from build123d import *

# Parameters (mm, degrees)
BOSS_EXTRUDE1_DEPTH          = 19.05
SKETCH7_R                    = 7.62
CUT_EXTRUDE2_DEPTH           = 38.1
SKETCH2_R                    = 11.176
CUT_EXTRUDE1_DEPTH           = 7.239
SKETCH8_R                    = 11.176
CUT_EXTRUDE3_DEPTH           = 7.239
F_10_0_1935_DIAMETER_HOLE1_D = 4.9149


with BuildPart() as part:
    # Sketch1 → Boss-Extrude1 (new body, symmetric)
    with BuildSketch(Plane.XY):
        Polygon((13.335, 25.4), (-13.335, 25.4), (-13.335, 38.1), (-20.447, 38.1), (-20.447, -71.12), (20.447, -71.12), (20.447, 38.1), (13.335, 38.1), align=None)
    extrude(amount=BOSS_EXTRUDE1_DEPTH, both=True)

    # Sketch7 → Cut-Extrude2 (cut)
    with BuildSketch(Plane.XY.offset(19.05)):
        Circle(SKETCH7_R)
        with Locations((0, -50.8)):
            Circle(SKETCH7_R)
    extrude(amount=-CUT_EXTRUDE2_DEPTH, mode=Mode.SUBTRACT)

    # Sketch2 → Cut-Extrude1 (cut)
    with BuildSketch(Plane.XY.offset(19.05)):
        Circle(SKETCH2_R)
        with Locations((0, -50.8)):
            Circle(SKETCH2_R)
    extrude(amount=-CUT_EXTRUDE1_DEPTH, mode=Mode.SUBTRACT)

    # Sketch8 → Cut-Extrude3 (cut)
    with BuildSketch(Plane.XY.offset(-19.05)):
        Circle(SKETCH8_R)
        with Locations((0, -50.8)):
            Circle(SKETCH8_R)
    extrude(amount=CUT_EXTRUDE3_DEPTH, mode=Mode.SUBTRACT)

    # #10 (0.1935) Diameter Hole1 (through all)
    with Locations(Plane(origin=(20.447, 0, 0), x_dir=(0, 0, -1), z_dir=(1, 0, 0))):
        with Locations((-11.43, 31.75)):
            f_10_0_1935_diameter_hole1 = Hole(F_10_0_1935_DIAMETER_HOLE1_D / 2)

    # Mirror1: #10 (0.1935) Diameter Hole1 across plane
    add(f_10_0_1935_diameter_hole1.mirror(Plane.XY), mode=Mode.SUBTRACT)


solid = part.part
For this review, take the finished solid that the model builds, in its own axes (mm). A direction names the side the tool comes from. Give positions to 0.01 mm unless a question says otherwise; leave off trailing zeros. Loops run counter-clockwise (first coordinate to the right, second up) from the corner with the lowest first, then second, coordinate; pieces in that order, holes last.
Item 1: Take a section at B-B, the plane z = -15.5. State the section outline as (x, y) points (3 decimals), and give its area (3 significant figures).
Item 2: Take a section at D-D, the plane y = 31.75. State the section outline as (x, z) points (3 decimals).
Item 3: Tool access review of faces 1 (the flat face through (0, -16, -19.05)), 2 (the cylindrical face through (-16.94, 33.41, -9.62)), 3 (the cylindrical face through (-1.45, -39.72, -15.48)), 4 (the cylindrical face through (-8.87, -6.8, 15.48)), 5 (the flat face through (-13.335, 32, 0)): name each direction out of +Z, -Z, +X, -X, +Y, -Y from which nothing blocks a thin tool from reaching the whole face with its end or side.
Item 4: Take a section at C-C, the plane y = -50.8. State the section outline as (x, z) points.
Item 5: For line 1 along Y through (x, z) = (0, -15.25); line 2 along Y through (x, z) = (18, 11.43); line 3 along X through (y, z) = (26, 16) (3 decimals), list the stretches that pass through material, from the lowest coordinate up.
Item 6: Draft analysis for pull direction Z (two halves, no side actions). For faces 6 (the flat face through (5, -7, 11.811)), 7 (the flat face through (-17, 38.1, 0)), 8 (the cylindrical face through (16.84, 33.41, 9.62)), state which applies: +Z half, -Z half, draft (parallel to the pull), parting line (faces both ways), or undercut.
Item 7: Insertion check: pin 1 (20 mm diameter, centred on x = 0, y = -50.8, fed in from -Z); pin 2 (4.5 mm diameter, centred on y = 31.75, z = 11.43, fed in from +X); pin 3 (21.5 mm diameter, centred on x = 2.5, z = -1.5, fed in from +Y); pin 4 (11 mm diameter, centred on x = -5, y = 1.5, fed in from +Z). Each pin has a flat end and moves straight along its axis. Give the tip position at first contact, or say it passes through.
Item 8: Take a section at A-A, the plane x = 0. State the section outline as (y, z) points, and give its area (3 significant figures).
Calculated:
1. outline: (-20.447, -71.12) - (20.447, -71.12) - (20.447, 38.1) - (13.335, 38.1) - (13.335, 25.4) - (-13.335, 25.4) - (-13.335, 38.1) - (-20.447, 38.1) - close; hole circle Ø22.352 at (0, -50.8); hole circle Ø22.352 at (0, 0)
1. area: 3,340 mm2
2. outline: (-20.447, -19.05) - (-13.335, -19.05) - (-13.335, -13.887) - (-20.447, -13.887) - close; (-20.447, -8.973) - (-13.335, -8.973) - (-13.335, 8.973) - (-20.447, 8.973) - close; (-20.447, 13.887) - (-13.335, 13.887) - (-13.335, 19.05) - (-20.447, 19.05) - close; (13.335, -19.05) - (20.447, -19.05) - (20.447, -13.887) - (13.335, -13.887) - close; (13.335, -8.973) - (20.447, -8.973) - (20.447, 8.973) - (13.335, 8.973) - close; (13.335, 13.887) - (20.447, 13.887) - (20.447, 19.05) - (13.335, 19.05) - close
3. face 1: -Z, +X, -X, +Y, -Y
3. face 2: +X, -X
3. face 3: -Z
3. face 4: +Z
3. face 5: +Z, -Z, +Y
4. outline: (-20.45, -19.05) - (-11.18, -19.05) - (-11.18, -11.81) - (-7.62, -11.81) - (-7.62, 11.81) - (-11.18, 11.81) - (-11.18, 19.05) - (-20.45, 19.05) - close; (7.62, -11.81) - (11.18, -11.81) - (11.18, -19.05) - (20.45, -19.05) - (20.45, 19.05) - (11.18, 19.05) - (11.18, 11.81) - (7.62, 11.81) - close
5. line 1: y = -71.12 to -61.98, -39.62 to -11.18, 11.18 to 25.4
5. line 2: y = -71.12 to 29.29, 34.21 to 38.1
5. line 3: x = -20.447 to -13.335, 13.335 to 20.447
6. face 6: +Z half
6. face 7: draft
6. face 8: undercut
7. pin 1: stops at z = -11.81
7. pin 2: passes through
7. pin 3: stops at y = 25.4
7. pin 4: stops at z = 11.81
8. outline: (-71.12, -19.05) - (-61.98, -19.05) - (-61.98, -11.81) - (-58.42, -11.81) - (-58.42, 11.81) - (-61.98, 11.81) - (-61.98, 19.05) - (-71.12, 19.05) - close; (-43.18, -11.81) - (-39.62, -11.81) - (-39.62, -19.05) - (-11.18, -19.05) - (-11.18, -11.81) - (-7.62, -11.81) - (-7.62, 11.81) - (-11.18, 11.81) - (-11.18, 19.05) - (-39.62, 19.05) - (-39.62, 11.81) - (-43.18, 11.81) - close; (7.62, -11.81) - (11.18, -11.81) - (11.18, -19.05) - (25.4, -19.05) - (25.4, 19.05) - (11.18, 19.05) - (11.18, 11.81) - (7.62, 11.81) - close
8. area: 2,310 mm2
